Geometry: final body of the model. Coordinates: model frame, mm. Face numbers are marked on the shaded views. Coordinates: 2 decimals unless noted, no trailing zeros. Order: outer loops, then holes, each group sorted by start corner. A loop starts at its lowest first (then second) coordinate and runs counter-clockwise, first axis right, second up. Notation, with made-up numbers: M 68,41 L 126,41 A20 ccw 126,76 Z; hole C 16.25,76 d2. An arc over 180 degrees is marked long. Use CSV: the item, a comma, the result in double quotes. Start each with the question number.
Q1. Section query C-C, the plane z = -72.5. Output: boundary loops of the cut face in (x, y) (3 decimals).
Q2. Section query D-D, the plane z = -19. Output: boundary loops of the cut face in (x, y).
Q3. Section query A-A, the plane y = 0. Output: boundary loops of the cut face in (x, z).
Q4. Mould query, pull axis X, two halves, no side actions, for the marked faces 1 and 2. Classes: +X half, -X half, draft (parallel to the pull), parting line (faces both ways), or undercut.
Q5. Ray query, probe 1 along X at (y, z) = (0, -119.2); probe 2 along X at (y, z) = (-21, -103.5); probe 3 along Y at (x, z) = (-48.5, -53). Return the intervals inside material, ascending.
Q6. First-contact query: P1, Ø1, axis at x = -56.5, z = -23.5, coming from the +Y side; P2, Ø1.5, axis at x = 14.5, z = -21.5, coming from the -Y side; P3, Ø4, axis at x = 0, y = 45, coming from the +Z side. Flat tips, straight axial feed; report the tip coordinate or a pass-through.
from build123d import *

# Parameters (mm, degrees)
F2_T     = -2
F3_DEPTH = 25


with BuildPart() as f1:
    # F0 (on Front) → F1 (revolve)
    with BuildSketch(Plane.XZ):
        Polygon((0, -120), (0, 0), (-80, 0), (-30, -120), align=None)
    revolve(axis=Axis((0, 0, -60), (0, 0, -1)))

    # F2
    f2_openings = [f1.faces().sort_by_distance(p)[0] for p in [
        (0, 0, 0),
    ]]
    offset(amount=F2_T, openings=f2_openings)

    # F3 (cut): a face of the model
    f3_faces = [f1.faces().sort_by_distance(p)[0] for p in [
        (0, 0, -118),
    ]]
    extrude(f3_faces, amount=-F3_DEPTH, mode=Mode.SUBTRACT)


solid = f1.part
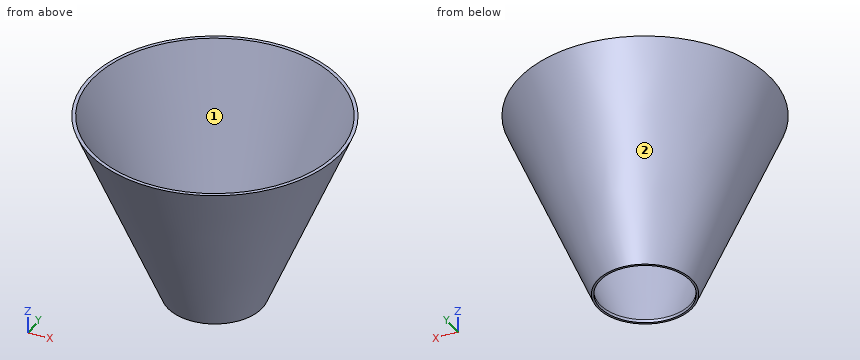
Responses:
1,outline,"C 0,0 d99.583; hole C 0,0 d95.25"
2,outline,"C 0,0 d144.17; hole C 0,0 d139.83"
3,outline,"M -80,0 L -30,-120 L -28.67,-120 L -28.67,-118 L -77.83,0 Z; M 28.67,-120 L 30,-120 L 80,0 L 77.83,0 L 28.67,-118 Z"
4,face 1,"undercut"
4,face 2,"parting line"
5,probe 1,"x = -30.33 to -28.67, 28.67 to 30.33"
5,probe 2,"x = -30.31 to -27.63, 27.63 to 30.31"
5,probe 3,"y = -31.66 to -27.49, 27.49 to 31.66"
6,P1,"stops at y = 42.43"
6,P2,"stops at y = -69.9"
6,P3,"stops at z = -74"
